The model under review builds one solid part; all positions refer to its coordinate system, in mm. Face numbers are marked on the shaded views. Coordinates: 2 decimals unless noted, no trailing zeros. Write each loop counter-clockwise with the first axis right and the second up, starting at its lowest first coordinate (ties: lowest second). Pieces come first, ordered by that corner, then holes. Notation, with made-up numbers: (1, -12.5) - (34, -12.5) arc R15 ccw to (34, 12.5) - close; hole circle Ø2 at (74.25, 66). An arc over 180 degrees is marked (long way). Put each result on its own line as item: value.
from build123d import *

# Parameters (mm, degrees)
SKETCH_W   = 31.75
SKETCH_H   = 31.75
SKETCH_W_2 = 26.2128
SKETCH_H_2 = 26.2128
PAD_DEPTH  = 546.1


with BuildPart() as part:
    # Sketch → Pad (new body)
    with BuildSketch(Plane.XZ):
        Rectangle(SKETCH_W, SKETCH_H)
        Rectangle(SKETCH_W_2, SKETCH_H_2, mode=Mode.SUBTRACT)
    extrude(amount=PAD_DEPTH)


solid = part.part
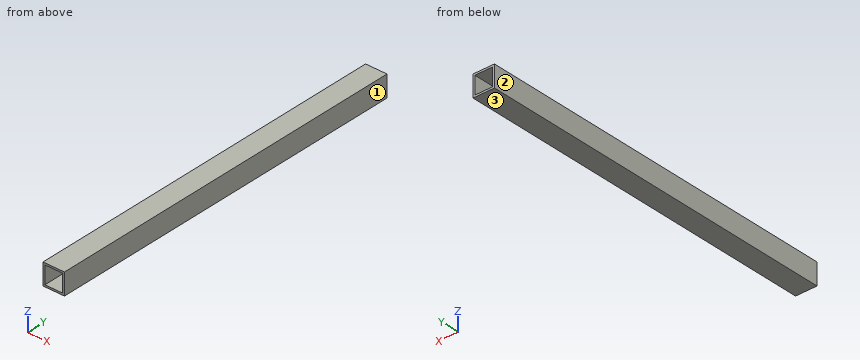
1. Consider section A-A on y = -363.5. State the section outline as (x, z) points (3 decimals), plus the area to 3 significant figures.
Determined:
outline: (-15.875, -15.875) - (15.875, -15.875) - (15.875, 15.875) - (-15.875, 15.875) - close; hole (-13.106, -13.106) - (13.106, -13.106) - (13.106, 13.106) - (-13.106, 13.106) - close
area: 321 mm^2
2. Consider section B-B on x = -5. State the section outline as (y, z) points (3 decimals), plus the area to 3 significant figures.
Determined:
outline: (-546.1, -15.875) - (0, -15.875) - (0, -13.106) - (-546.1, -13.106) - close; (-546.1, 13.106) - (0, 13.106) - (0, 15.875) - (-546.1, 15.875) - close
area: 3,020 mm^2
3. To check wall thickness, follow probe 1 along X at (y, z) = (-168, -5) (3 decimals). State the ranges of the line that lie inside material, in increasing order.
Determined:
probe 1: x = -15.875 to -13.106, 13.106 to 15.875
4. Consider section C-C on z = -5.5. State the section outline as (x, y) points (3 decimals).
Determined:
outline: (-15.875, -546.1) - (-13.106, -546.1) - (-13.106, 0) - (-15.875, 0) - close; (13.106, -546.1) - (15.875, -546.1) - (15.875, 0) - (13.106, 0) - close
5. The part is to be moulded in two halves that separate along X. For the marked faces 1, 2 and 3, say which applies: +X half, -X half, draft (parallel to the pull), parting line (faces both ways), or undercut.
Determined:
face 1: +X half
face 2: -X half
face 3: draft
